```python
from build123d import *

# Parameters (mm, degrees)
SKETCH1_R           = 1.975
BOSS_EXTRUDE1_DEPTH = 4.5


with BuildPart() as part:
    # Sketch1 → Boss-Extrude1 (new body)
    with BuildSketch(Plane(origin=(0, 0, 0), x_dir=(1, 0, 0), z_dir=(0, 1, 0))):
        with BuildLine():
            Line((30.5816, 20.675), (-30.5816, 20.675))
            ThreePointArc((-30.5816, 20.675), (-32.377651224, 19.931051224), (-33.1216, 18.135))
            Line((-33.1216, 18.135), (-33.1216, -18.135))
            ThreePointArc((-33.1216, -18.135), (-32.377651224, -19.931051224), (-30.5816, -20.675))
            Line((-30.5816, -20.675), (-13.187240763, -20.675))
            ThreePointArc((-13.187240763, -20.675), (-12.081828105, -20.421845613), (-11.196761955, -19.712844768))
            add(Edge.make_bspline(
                [(11.196761955, -19.712844768), (8.939286543, -16.865), (0, -16.865), (-8.939286543, -16.865), (-11.196761955, -19.712844768)],
                knots=[3.396891088, 3.396891088, 3.396891088, 4.71238898, 4.71238898, 6.027886873, 6.027886873, 6.027886873], degree=2, weights=[1, 0.791370388, 1, 0.791370388, 1]))
            ThreePointArc((11.196761955, -19.712844768), (12.081828105, -20.421845613), (13.187240763, -20.675))
            Line((13.187240763, -20.675), (30.5816, -20.675))
            ThreePointArc((30.5816, -20.675), (32.377651224, -19.931051224), (33.1216, -18.135))
            Line((33.1216, -18.135), (33.1216, 18.135))
            ThreePointArc((33.1216, 18.135), (32.377651224, 19.931051224), (30.5816, 20.675))
        make_face()
        with Locations(Location((-20.8153, 0, 0), (0, 0, 270))):
            Circle(SKETCH1_R, mode=Mode.SUBTRACT)
        with Locations(Location((20.8153, 0, 0), (0, 0, 90))):
            Circle(SKETCH1_R, mode=Mode.SUBTRACT)
    extrude(amount=BOSS_EXTRUDE1_DEPTH)


solid = part.part
```
Here's how the part is built. I have some questions about the finished solid (model axes, mm). A direction names the side the tool comes from. Give positions to 0.01 mm unless a question says otherwise; leave off trailing zeros. Order: outer loops, then holes, each group sorted by start corner. A loop starts at its lowest first (then second) coordinate and runs counter-clockwise, first axis right, second up. Notation, with made-up numbers: (-10.75, -31.75) -> (43.25, -31.75) arc R29 cw to (43.25, -9.75) -> close; hole circle Ø3 at (88.25, 52). An arc over 180 degrees is marked (long way). Use CSV: the item, a comma, the result in double quotes. Start each with the question number.
Item 1: If I drill on probe 1 along X at (y, z) = (3.1, 0); probe 2 along X at (y, z) = (3.35, -1); probe 3 along Z at (x, y) = (-4, 0.25) (3 decimals), over which ranges is the centre line in solid material (lowest first)? Write a range as [from, to].
Item 2: Suppose I cut it at B-B (y = 1). Give the number of separate pieces and of enclosed holes in the cut face, and give its area (3 significant figures).
Item 3: Suppose I cut it at A-A (z = 0). List the corners of the cut face in (x, y) for me.
Item 4: On a 3-axis mill with a long thin cutter (end or side, diameter ignored), from which of +Z, -Z, +X, -X, +Y, -Y can I reach the whole of each face in a straight line? I mean faces 1 (the flat face through (-33.122, 2, 0)), 2 (the cylindrical face through (-12.1, 2.22, 20.43)). Say none if no direction works.
Item 5: I'm going to push a flat-ended pin straight in: P1, Ø1, axis at x = -6.5, y = 2.5, coming from the +Z side. Where does the tip first touch, or does it pass through?
Item 6: Thinking about a two-plate mould opening in X: for faces 3 (the cylindrical face through (32.4, 2.22, -19.91)), 4 (the cylindrical face through (-32.4, 2.22, 19.91)), 5 (the flat face through (0, 2, -20.675)), 6 (the cylindrical face through (-22.017, 2.218, -1.567)), which applies, pulls with the +X half, pulls with the -X half, needs draft (parallel to the pull), parting line crosses it, or undercut?
Answer block:
1,probe 1,"x = [-33.12, -22.79], [-18.84, 18.84], [22.79, 33.12]"
1,probe 2,"x = [-33.12, -22.52], [-19.11, 19.11], [22.52, 33.12]"
1,probe 3,"z = [-20.675, 17.1]"
2,separate pieces,"1"
2,enclosed holes,"2"
2,area,"2,640 mm^2"
3,outline,"(-33.12, 0) -> (-22.79, 0) -> (-22.79, 4.5) -> (-33.12, 4.5) -> close; (-18.84, 0) -> (18.84, 0) -> (18.84, 4.5) -> (-18.84, 4.5) -> close; (22.79, 0) -> (33.12, 0) -> (33.12, 4.5) -> (22.79, 4.5) -> close"
4,face 1,"+Z, -Z, -X, +Y, -Y"
4,face 2,"+Z, +Y, -Y"
5,P1,"stops at z = 17.64"
6,face 3,"pulls with the +X half"
6,face 4,"pulls with the -X half"
6,face 5,"needs draft"
6,face 6,"undercut"
